Build history of the part. All positions in model axes, mm. A direction names the side the tool comes from. Give positions to 0.01 mm unless a question says otherwise; leave off trailing zeros. Order: outer loops, then holes, each group sorted by start corner. A loop starts at its lowest first (then second) coordinate and runs counter-clockwise, first axis right, second up. Notation, with made-up numbers: (36.25, -25) - (42.25, -25) arc R31 ccw to (42.25, 6) - close; hole circle Ø8 at (41.25, -26). An arc over 180 degrees is marked (long way). Write each question's results on one line, items separated by ' | '. Start each with the question number.
1) Two-plate mould, pull along Y, no slides. Class faces 1 (the face through (5, -4, -60)), 2 (the face through (5, 300, -1)), 3 (the face through (5, -4, 37.5)): +Y half, -Y half, draft (parallel to the pull), parting line (faces both ways), or undercut.
2) Drill centre lines: line 1 along Y through (x, z) = (7.75, 9); line 2 along Z through (x, y) = (5.25, 11). Where is each one in solid material? Low to high. Write a range as from..to.
3) Cut at A-A on y = 173.5. List the corners of the cut face in (x, z), plus the area to 3 significant figures.
4) Cut at C-C on z = 4.5. List the corners of the cut face in (x, y), plus the area to 3 significant figures.
5) Cut at B-B on x = 4.5. List the corners of the cut face in (y, z), plus the area to 3 significant figures.
6) Tool access for faces 4 (the face through (10, -4, 41)), 5 (the face through (5, -4, -37.5)): list every direction of +Z, -Z, +X, -X, +Y, -Y with a clear straight run to the whole face (end or side of a thin tool).
from build123d import *

# Parameters (mm, degrees)
SKETCH_W     = 600
SKETCH_H     = 120
PAD_DEPTH    = 10
SKETCH001_W  = 540
SKETCH001_H  = 75
POCKET_DEPTH = 10


with BuildPart() as part:
    # Sketch → Pad (new body)
    with BuildSketch(Plane.YZ):
        Rectangle(SKETCH_W, SKETCH_H)
    extrude(amount=PAD_DEPTH)

    # Sketch001 → Pocket (cut)
    with BuildSketch(Plane.YZ.offset(10)):
        Rectangle(SKETCH001_W, SKETCH001_H)
    extrude(amount=-POCKET_DEPTH, mode=Mode.SUBTRACT)


solid = part.part
Results:
1) face 1: draft | face 2: +Y half | face 3: undercut
2) line 1: -300..-270, 270..300 | line 2: -60..-37.5, 37.5..60
3) outline: (0, -60) - (10, -60) - (10, -37.5) - (0, -37.5) - close; (0, 37.5) - (10, 37.5) - (10, 60) - (0, 60) - close | area: 450 mm^2
4) outline: (0, -300) - (10, -300) - (10, -270) - (0, -270) - close; (0, 270) - (10, 270) - (10, 300) - (0, 300) - close | area: 600 mm^2
5) outline: (-300, -60) - (300, -60) - (300, 60) - (-300, 60) - close; hole (-270, -37.5) - (270, -37.5) - (270, 37.5) - (-270, 37.5) - close | area: 31,500 mm^2
6) face 4: +Z, -Z, +X, +Y, -Y | face 5: +X, -X
